from build123d import *

# Parameters (mm, degrees)
SKETCH2_W           = 120.65
SKETCH2_H           = 120.65
BOSS_EXTRUDE1_DEPTH = 2.54
SKETCH3_W           = 23.495
SKETCH3_H           = 6.35
SKETCH3_W_2         = 52.07
SKETCH3_W_3         = 109.22
SKETCH3_H_2         = 27.94
SKETCH3_W_4         = 0.635
SKETCH3_H_3         = 38.1
SKETCH3_H_4         = 16.51
BOSS_EXTRUDE2_DEPTH = 2.54
BOSS_EXTRUDE4_DEPTH = 2.54


with BuildPart() as part:
    # Sketch2 → Boss-Extrude1 (new body)
    with BuildSketch(Plane(origin=(0, 0, 0), x_dir=(1, 0, 0), z_dir=(0, 1, 0))):
        Rectangle(SKETCH2_W, SKETCH2_H)
    extrude(amount=BOSS_EXTRUDE1_DEPTH)

    # Sketch3 → Boss-Extrude2 (add)
    with BuildSketch(Plane(origin=(0, 2.54, 0), x_dir=(1, 0, 0), z_dir=(0, 1, 0))):
        with Locations((-42.8625, -21.59)):
            Rectangle(SKETCH3_W, SKETCH3_H)
        with Locations((0, -21.59)):
            Rectangle(SKETCH3_W_2, SKETCH3_H)
        with Locations((42.8625, -21.59)):
            Rectangle(SKETCH3_W, SKETCH3_H)
        with Locations((0, -46.355)):
            Rectangle(SKETCH3_W_3, SKETCH3_H_2)
        with Locations((-60.0075, 5.715)):
            Rectangle(SKETCH3_W_4, SKETCH3_H_3)
        with Locations((-60.0075, 35.56)):
            Rectangle(SKETCH3_W_4, SKETCH3_H)
        with Locations((-60.0075, 52.07)):
            Rectangle(SKETCH3_W_4, SKETCH3_H_4)
        with Locations((60.0075, 52.07)):
            Rectangle(SKETCH3_W_4, SKETCH3_H_4)
        with Locations((60.0075, 35.56)):
            Rectangle(SKETCH3_W_4, SKETCH3_H)
        with Locations((60.0075, 5.715)):
            Rectangle(SKETCH3_W_4, SKETCH3_H_3)
        with Locations((-60.0075, -21.59)):
            Rectangle(SKETCH3_W_4, SKETCH3_H)
        with Locations((60.0075, -21.59)):
            Rectangle(SKETCH3_W_4, SKETCH3_H)
        with Locations((60.0075, -46.355)):
            Rectangle(SKETCH3_W_4, SKETCH3_H_2)
        with Locations((-60.0075, -46.355)):
            Rectangle(SKETCH3_W_4, SKETCH3_H_2)
        with Locations((-42.8625, 35.56)):
            Rectangle(SKETCH3_W, SKETCH3_H)
        with Locations((0, 35.56)):
            Rectangle(SKETCH3_W_2, SKETCH3_H)
        with Locations((42.8625, 35.56)):
            Rectangle(SKETCH3_W, SKETCH3_H)
        with Locations((0, 52.07)):
            Rectangle(SKETCH3_W_3, SKETCH3_H_4)
        with Locations((0, 5.715)):
            Rectangle(SKETCH3_W_3, SKETCH3_H_3)
    extrude(amount=BOSS_EXTRUDE2_DEPTH)

    # Sketch5 → Boss-Extrude4 (add)
    with BuildSketch(Plane(origin=(60.325, 0, 0), x_dir=(0, 0, -1), z_dir=(1, 0, 0))):
        Polygon((-60.325, 0), (60.325, 0), (60.325, 5.08), (43.815, 5.08), (43.815, 2.54), (38.735, 2.54), (38.735, 5.08), (32.385, 5.08), (32.385, 2.54), (24.765, 2.54), (24.765, 5.08), (-13.335, 5.08), (-13.335, 2.54), (-18.415, 2.54), (-18.415, 5.08), (-24.765, 5.08), (-24.765, 2.54), (-32.385, 2.54), (-32.385, 5.08), (-60.325, 5.08), align=None)
    boss_extrude4 = extrude(amount=BOSS_EXTRUDE4_DEPTH)

    # Mirror2: Boss-Extrude4 across plane
    add(boss_extrude4.mirror(Plane(origin=(0, 0, 0), x_dir=(0, 0, 1), z_dir=(1, 0, 0))))


solid = part.part
Design review of the part built by this model. Coordinates are the model's own, in mm. Give positions to 0.01 mm unless a question says otherwise; leave off trailing zeros. Loops run counter-clockwise (first coordinate to the right, second up) from the corner with the lowest first, then second, coordinate; pieces in that order, holes last. Notation, with made-up numbers: M 46.25,-33 L 86.25,-33 A37 ccw 86.25,3 Z; hole C 18,75.5 d2. An arc over 180 degrees is marked long. Answer as a JSON object with one key per item and string values.
Item 1: We need section A-A (z = 8.5). State the section outline as (x, y) points (3 decimals).
Output values:
{"outline": "M -62.865,0 L 62.865,0 L 62.865,5.08 L 59.69,5.08 L 59.69,2.54 L 54.61,2.54 L 54.61,5.08 L -54.61,5.08 L -54.61,2.54 L -59.69,2.54 L -59.69,5.08 L -62.865,5.08 Z"}
Item 2: We need section C-C (y = 3.95). Count the separate pieces of the cut face and the enclosed holes in it, and give its area (3 significant figures).
Output values:
{"separate pieces": "19", "enclosed holes": "0", "area": "10,900 mm2"}
Item 3: Wall thickness on line 1 along X through (y, z) = (4.4, 38) (3 decimals); line 2 along Z through (x, y) = (50.5, 4.15) (3 decimals); line 3 along Z through (x, y) = (-29.5, 4.2) (3 decimals): over which ranges is each line inside the solid? List them lowest first.
Output values:
{"line 1": "x = -62.865 to -59.69, -54.61 to 54.61, 59.69 to 62.865", "line 2": "z = -60.325 to -43.815, -38.735 to -32.385, -24.765 to 13.335, 18.415 to 24.765, 32.385 to 60.325", "line 3": "z = -60.325 to -43.815, -24.765 to 13.335, 32.385 to 60.325"}
Item 4: Mouldability with a two-part tool opening along X and no side actions: class faces 1 (the face through (-61, 5.08, -52)), 2 (the face through (-62.865, 2, 1)), 3 (the face through (1, 2.54, -28)) as pulls with the +X half, pulls with the -X half, needs draft (parallel to the pull), parting line crosses it, or undercut.
Output values:
{"face 1": "needs draft", "face 2": "pulls with the -X half", "face 3": "undercut"}
Item 5: We need section B-B (x = -15). State the section outline as (y, z) points (3 decimals), and give its area (3 significant figures).
Output values:
{"outline": "M 0,-60.325 L 5.08,-60.325 L 5.08,-43.815 L 2.54,-43.815 L 2.54,-38.735 L 5.08,-38.735 L 5.08,-32.385 L 2.54,-32.385 L 2.54,-24.765 L 5.08,-24.765 L 5.08,13.335 L 2.54,13.335 L 2.54,18.415 L 5.08,18.415 L 5.08,24.765 L 2.54,24.765 L 2.54,32.385 L 5.08,32.385 L 5.08,60.325 L 0,60.325 Z", "area": "548 mm2"}
